Could you check a few things on this model? Use its own coordinates, in mm. Round coordinates to 2 decimals unless told otherwise and drop trailing zeros. Loops run counter-clockwise (first coordinate to the right, second up) from the corner with the lowest first, then second, coordinate; pieces in that order, holes last. Notation, with made-up numbers: (65.25, 24.25) -> (110.25, 24.25) arc R27 ccw to (110.25, 43.25) -> close; hole circle Ø4 at (10.5, 46). An arc over 180 degrees is marked (long way). One line per item, written item: value.
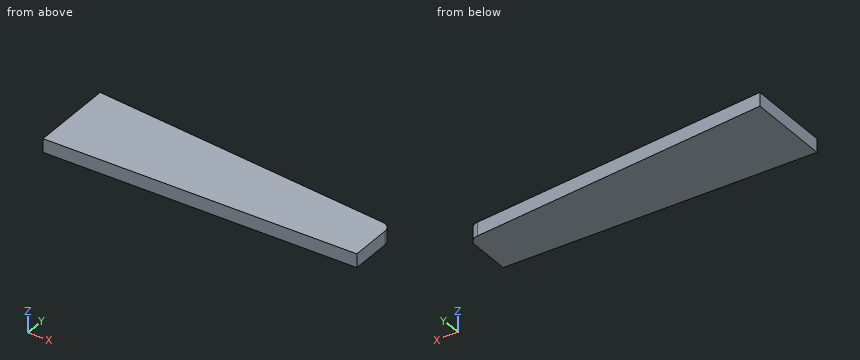
Autodesk Inventor part; units mm, degrees
ref_plane "YZ Plane" through (0, 0, 0) normal (1, 0, 0) x (0, 1, 0)
ref_plane "XZ Plane" through (0, 0, 0) normal (0, 1, 0) x (-1, 0, 0)
ref_plane "XY Plane" through (0, 0, 0) normal (0, 0, 1) x (1, 0, 0)
sketch "Sketch3" plane through (0, 0, 0) normal (0, 0, 1) x (1, 0, 0)
  line L0 (0, 0) -> (230, 0)
  line L1 (230, 0) -> (230, 30)
  line L2 (230, 30) -> (-74.7049, 62.9411)
  line L3 (45, 50) -> (45, 0)
  dimension "d11" = 230
  dimension "d12" = 30
  dimension "d13" = 45
  dimension "d14" = 50
extrude "Plate1" add sketch "Sketch3" along normal mid plane 8
fillet "Corner Round1" radius 6 1 edges at (230, 30, 0)
equation "\"d15\" = Thickness"
equation "\"BendRadius\" = Thickness"
equation "\"BendReliefWidth\" = Thickness"
equation "\"BendReliefDepth\" = 0.5 * Thickness"
equation "\"CornerReliefSize\" = 4 * Thickness"
equation "\"MinimumRemnant\" = 2 * Thickness"
equation "\"TransitionRadius\" = BendRadius"
equation "\"JacobiRadiusSize\" = BendRadius"
equation "\"GapSize\" = Thickness"
properties part number "APN 1413 charging hatch reinf" material "Steel"
Item 1: If we section it at C-C on y = 43: List the corners of the cut face in (x, z) for me.
Output:
outline: (45, -4) -> (109.75, -4) -> (109.75, 4) -> (45, 4) -> close
Item 2: If we section it at B-B on x = 57.5: List the corners of the cut face in (y, z) for me, plus the area to 3 significant figures.
Output:
outline: (0, -4) -> (48.65, -4) -> (48.65, 4) -> (0, 4) -> close
area: 389 mm²
Item 3: I need wall thicknesses on line 1 (Y direction, x = 218.5, z = -0.25); line 2 (Y direction, x = 213.5, z = 0.5); line 3 (X direction, y = 29.5, z = -1). Which ranges of each line are inside material? Lowest first, please. Write a range as from..to.
Output:
line 1: y = 0..31.24
line 2: y = 0..31.78
line 3: x = 45..227.48
Item 4: If we section it at A-A on z = 1.25: List the corners of the cut face in (x, y) for me, plus the area to 3 significant figures.
Output:
outline: (45, 0) -> (230, 0) -> (230, 24.61) arc R6 ccw to (224.64, 30.58) -> (45, 50) -> close
area: 7,390 mm²
